from build123d import *

# Parameters (mm, degrees)
SKETCH1_W            = 90
SKETCH1_H            = 65
SKETCH1_R            = 2.875
BOSS_EXTRUDE1_DEPTH  = 1
FILLET1_R            = 10
BOSS_EXTRUDE2_START  = -37
SKETCH2_R            = 2
BOSS_EXTRUDE2_DEPTH  = 1
FILLET2_R            = 6
FILLET2_OF_MIRROR1_R = 6


with BuildPart() as part:
    # Sketch1 → Boss-Extrude1 (new body)
    with BuildSketch(Plane(origin=(0, 0, 0), x_dir=(1, 0, 0), z_dir=(0, 1, 0))):
        Rectangle(SKETCH1_W, SKETCH1_H)
        with Locations((-36.375, 23.875)):
            Circle(SKETCH1_R, mode=Mode.SUBTRACT)
        with Locations((36.375, 23.875)):
            Circle(SKETCH1_R, mode=Mode.SUBTRACT)
        with Locations((36.375, -23.875)):
            Circle(SKETCH1_R, mode=Mode.SUBTRACT)
        with Locations((-36.375, -23.875)):
            Circle(SKETCH1_R, mode=Mode.SUBTRACT)
    extrude(amount=BOSS_EXTRUDE1_DEPTH)

    # Fillet1
    fillet1_edges = [part.edges().sort_by_distance(p)[0] for p in [
        (45, 0.5, 32.5),
        (-45, 0.5, 32.5),
        (-45, 0.5, -32.5),
        (45, 0.5, -32.5),
    ]]
    fillet(fillet1_edges, radius=FILLET1_R)

    # Sketch2 → Boss-Extrude2 (add)
    with BuildSketch(Plane(origin=(45, 0, 0), x_dir=(0, 0, -1), z_dir=(1, 0, 0)).offset(BOSS_EXTRUDE2_START)):
        Polygon((-12.5, 1), (-10, 27), (10, 27), (12.5, 1), align=None)
        with Locations((0, 21)):
            Circle(SKETCH2_R, mode=Mode.SUBTRACT)
    boss_extrude2 = extrude(amount=-BOSS_EXTRUDE2_DEPTH)

    # Fillet2
    fillet2_edges = [part.edges().sort_by_distance(p)[0] for p in [
        (7.5, 27, 10),
        (7.5, 27, -10),
    ]]
    fillet(fillet2_edges, radius=FILLET2_R)

    # Mirror1: Boss-Extrude2 across plane
    add(boss_extrude2.mirror(Plane.ZY))

    # Fillet2 of Mirror1
    fillet2_of_mirror1_edges = [part.edges().sort_by_distance(p)[0] for p in [
        (-7.5, 27, 10),
        (-7.5, 27, -10),
    ]]
    fillet(fillet2_of_mirror1_edges, radius=FILLET2_OF_MIRROR1_R)


solid = part.part
Source: CAD feature listing. Evaluate the final solid. Frame: model axes, mm. A direction names the side the tool comes from. Round coordinates to 2 decimals unless told otherwise and drop trailing zeros. Loops run counter-clockwise (first coordinate to the right, second up) from the corner with the lowest first, then second, coordinate; pieces in that order, holes last. Notation, with made-up numbers: M 61,53 L 99,53 A22 cw 99,83 Z; hole C 78.5,-38 d3. An arc over 180 degrees is marked long. Return JSON: item names as keys, results as strings. Group by question number.
1. Section query C-C on y = 17.75. Output: boundary loops of the cut face in (x, z), and give its area (3 significant figures).
2. Mould query, pull axis Y, two halves, no side actions, for faces 1 (the face through (7.507, 11.143, 11.525)), 2 (the face through (-37, 0.49, -21.07)), 3 (the face through (-7.507, 22.983, 0.26)). Classes: released by +Y, released by -Y, zero draft, split by the parting line, or undercut.
3. Section query A-A on y = 25. Output: boundary loops of the cut face in (x, z), and give its area (3 significant figures).
4. Section query D-D on x = 2. Output: boundary loops of the cut face in (y, z).
5. Pin query (flat end, axial travel): pin 1 (7.5 mm diameter, centred on y = 15, z = -4, fed in from +X); pin 2 (4 mm diameter, centred on x = 3, z = 12, fed in from +Y). Return the tip coordinate at first contact, or that it passes through.
6. Section query B-B on z = 0. Output: boundary loops of the cut face in (x, y).
7. Reachability of faces 4 (the face through (-37, 0.49, 26.68)), 5 (the face through (7, 14, 0)), 6 (the face through (-8, 14, 0)) from +Z, -Z, +X, -X, +Y, -Y: full face, straight path, thin tool, end or side. Return the list, or none.
8. Material intervals for line 1 along X through (y, z) = (1.25, 3); line 2 along Y through (x, z) = (-2, 21), sorted ascending. Write a range as from..to.
Checks:
{
 "1": {"outline": "M -8,-10.89 L -7,-10.89 L -7,10.89 L -8,10.89 Z; M 7,-10.89 L 8,-10.89 L 8,10.89 L 7,10.89 Z", "area": "43.6 mm²"},
 "2": {"face 1": "released by +Y", "face 2": "zero draft", "face 3": "undercut"},
 "3": {"outline": "M -8,-9.02 L -7,-9.02 L -7,9.02 L -8,9.02 Z; M 7,-9.02 L 8,-9.02 L 8,9.02 L 7,9.02 Z", "area": "36.1 mm²"},
 "4": {"outline": "M 0,-32.5 L 1,-32.5 L 1,32.5 L 0,32.5 Z"},
 "5": {"pin 1": "stops at x = 8", "pin 2": "stops at y = 1"},
 "6": {"outline": "M -45,0 L 45,0 L 45,1 L 8,1 L 8,19 L 7,19 L 7,1 L -7,1 L -7,19 L -8,19 L -8,1 L -45,1 Z; M -8,23 L -7,23 L -7,27 L -8,27 Z; M 7,23 L 8,23 L 8,27 L 7,27 Z"},
 "7": {"face 4": "+Y, -Y", "face 5": "+Z, -Z, +Y", "face 6": "+Z, -Z, -X, +Y"},
 "8": {"line 1": "x = -8..-7, 7..8", "line 2": "y = 0..1"}
}
